Print and shaded views of the part. All mm, measured from the part's lowest x, y and z. Give positions to 0.01 mm unless a question says otherwise; leave off trailing zeros. Loops run counter-clockwise (first coordinate to the right, second up) from the corner with the lowest first, then second, coordinate; pieces in that order, holes last. Notation, with made-up numbers: M -17.5,86 L -0.5,86 A29 ccw -0.5,122 Z; hole C 67,47 d9. An arc over 180 degrees is marked long. Answer as CSV lines item,"result".
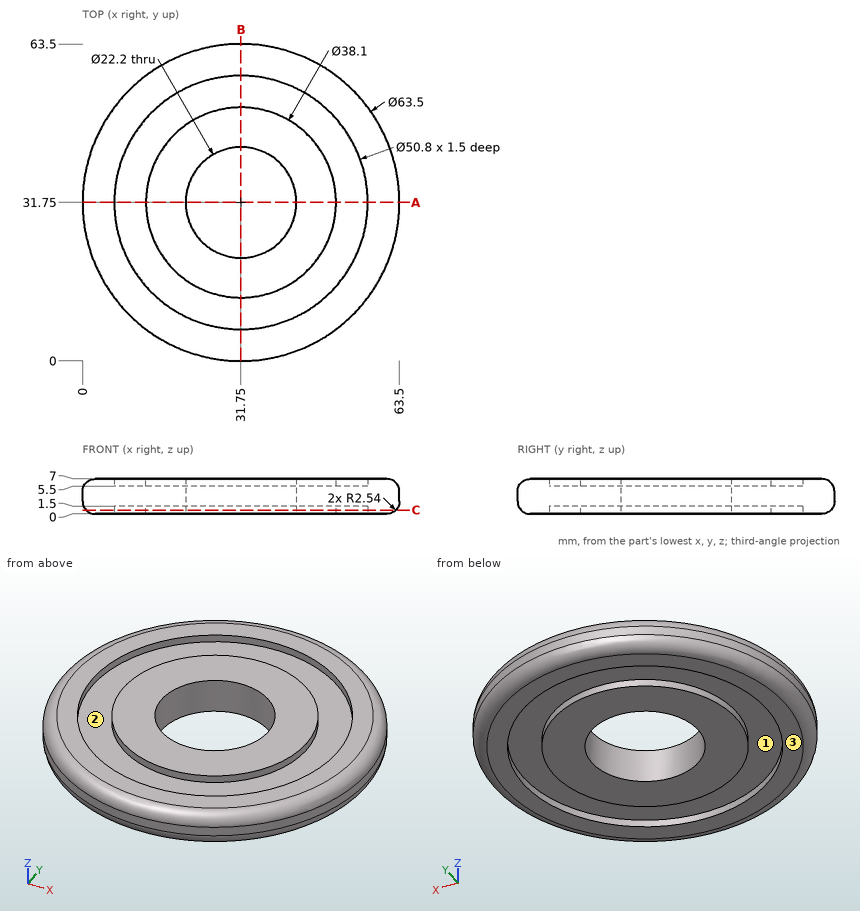
Q1. Cut at A-A (y = 31.75). Write the cut outline in (x, z), and give its area (3 significant figures).
Solution:
outline,"M 0,2.54 A2.54 ccw 2.54,0 L 6.35,0 L 6.35,1.5 L 12.7,1.5 L 12.7,0 L 20.65,0 L 20.65,7 L 12.7,7 L 12.7,5.5 L 6.35,5.5 L 6.35,7 L 2.54,7 A2.54 ccw 0,4.46 Z; M 42.85,0 L 50.8,0 L 50.8,1.5 L 57.15,1.5 L 57.15,0 L 60.96,0 A2.54 ccw 63.5,2.54 L 63.5,4.46 A2.54 ccw 60.96,7 L 57.15,7 L 57.15,5.5 L 50.8,5.5 L 50.8,7 L 42.85,7 Z"
area,"245 mm²"
Q2. Cut at C-C (z = 0.75). Write the cut outline in (x, y).
Solution:
outline,"C 31.75,31.75 d62.02; C 31.75,31.75 d38.1; hole C 31.75,31.75 d50.8; hole C 31.75,31.75 d22.2"
Q3. Pin check, flat tips, straight feed: P1, Ø4, axis at y = 23.5, z = 2, coming from the -X side; P2, Ø5, axis at x = 23, y = 53, coming from the -Z side; P3, Ø1, axis at x = 34, z = 4.5, coming from the -Y side; P4, Ø4, axis at y = 37, z = 4.5, coming from the +X side. Stop position of each tip, or through.
Solution:
P1,"stops at x = 0.63"
P2,"stops at z = 0"
P3,"stops at y = 0.05"
P4,"stops at x = 63.33"
Q4. Wall check: line 1 (X direction, y = 23.5, z = 0.5); line 2 (Y direction, x = 31.75, z = 0.4); line 3 (X direction, y = 41, z = 0.75). Give the ranges that are in metal, low to high. Write a range as [from, to].
Solution:
line 1,"x = [2.16, 7.73], [14.58, 24.32], [39.18, 48.92], [55.77, 61.34]"
line 2,"y = [1.17, 6.35], [12.7, 20.65], [42.85, 50.8], [57.15, 62.33]"
line 3,"x = [2.15, 8.09], [15.1, 25.61], [37.89, 48.4], [55.41, 61.35]"
Q5. Mould opens along Y. For the marked faces 1, 2 and 3 say: released by +Y, released by -Y, zero draft, split by the parting line, or undercut.
Solution:
face 1,"undercut"
face 2,"undercut"
face 3,"zero draft"
